Input: part model. Units: mm. Frame: model coordinates. A direction names the side the tool comes from. Round coordinates to 2 decimals unless told otherwise and drop trailing zeros. Write each loop counter-clockwise with the first axis right and the second up, starting at its lowest first coordinate (ties: lowest second). Pieces come first, ordered by that corner, then holes. Notation, with made-up numbers: (-6.5, 45.5) -> (11.5, 45.5) arc R18 ccw to (11.5, 57.5) -> close; hole circle Ø8 at (26.5, 40). An arc over 180 degrees is marked (long way). Write item = value, one per line.
```python
from build123d import *

# Parameters (mm, degrees)
F2_R = 7.5


with BuildPart() as f3:
    # F3: sweep along a path in F0
    with BuildLine(Plane.XZ) as f3_path:
        Line((13.8293646224, 0), (42.5, 0))
        Line((42.5, 0), (42.5, 72.5))
        ThreePointArc((42.5, 72.5), (30.0520382004, 102.5520382004), (0, 115))
        ThreePointArc((0, 115), (-30.0520382004, 102.5520382004), (-42.5, 72.5))
        Line((-42.5, 72.5), (-42.5, 0))
        Line((-42.5, 0), (-13.8293646224, 0))
    # F2 (on plane+point) → F3 (sweep)
    with BuildSketch(Plane.YZ.offset(-13.8293646224)):
        Circle(F2_R)
    sweep(path=f3_path.line, transition=Transition.RIGHT)


solid = f3.part
```
1) Line query: L1, parallel to X at y = 0.25, z = 57; L2, parallel to Z at x = -29, y = -5.75; L3, parallel to Z at x = 14, y = 1.5. Output: solid intervals per line, ascending. Write a range as from..to.
Solutions:
L1 = -50..-35, 35..50
L2 = -4.82..4.82, 96.57..109.89
L3 = -7.35..7.35, 104.74..120.34
2) Cut plane D-D (z = 52). Return the cut outline in (x, y), and give its area (3 significant figures).
Solutions:
outline = circle Ø15 at (-42.5, 0); circle Ø15 at (42.5, 0)
area = 353 mm^2
3) First-contact query: P1, Ø10, axis at x = -3.5, z = 109.5, coming from the +Y side; P2, Ø3, axis at x = 30, y = 0.5, coming from the +Z side; P3, Ø4, axis at x = 33.5, y = 1.5, coming from the -Z side; P4, Ø2, axis at x = -36.5, y = 1, coming from the +Z side. Flat tips, straight axial feed; report the tip coordinate or a pass-through.
Solutions:
P1 = 7.49
P2 = 113.57
P3 = -7.5
P4 = 107.63
4) Access query for faces 1 (the face through (-49.82, -1.63, 31.94)), 2 (the face through (-13.829, 0, 0)). Directions: +Z, -Z, +X, -X, +Y, -Y. A direction counts if a zero-diameter tool reaches every point of the face in a straight line with its end or side. Return the directions, or none.
Solutions:
face_1 = none
face_2 = -Z, +Y, -Y
5) Draft query along X for faces 3 (the face through (13.829, 0, 0)), 4 (the face through (-27.64, -1.63, -7.32)). Return one class per face: +X half, -X half, draft (parallel to the pull), parting line (faces both ways), or undercut.
Solutions:
face_3 = undercut
face_4 = undercut
6) Cut plane A-A (y = 6). Return the cut outline in (x, z).
Solutions:
outline = (-47, -4.5) -> (-13.83, -4.5) -> (-13.83, 4.5) -> (-38, 4.5) -> (-38, 72.5) arc R38 cw to (38, 72.5) -> (38, 4.5) -> (13.83, 4.5) -> (13.83, -4.5) -> (47, -4.5) -> (47, 72.5) arc R47 ccw to (-47, 72.5) -> close
7) Cut plane C-C (y = 0). Return the cut outline in (x, z), and give its area (3 significant figures).
Solutions:
outline = (-50, -7.5) -> (-13.83, -7.5) -> (-13.83, 7.5) -> (-35, 7.5) -> (-35, 72.5) arc R35 cw to (35, 72.5) -> (35, 7.5) -> (13.83, 7.5) -> (13.83, -7.5) -> (50, -7.5) -> (50, 72.5) arc R50 ccw to (-50, 72.5) -> close
area = 5,040 mm^2
8) Cut plane B-B (z = 5). Return the cut outline in (x, y).
Solutions:
outline = (-37.5, -5.59) -> (-13.83, -5.59) -> (-13.83, 5.59) -> (-37.5, 5.59) arc R7.5 ccw (long way) to start; (13.83, -5.59) -> (37.5, -5.59) arc R7.5 ccw (long way) to (37.5, 5.59) -> (13.83, 5.59) -> close
